Autodesk Inventor part; units mm, degrees
ref_plane "Arbeitsebene13" through (0, 0, 0) normal (0, 0, 1) x (1, 0, 0)
ref_plane "YZ Plane" through (0, 0, 0) normal (1, 0, 0) x (0, 1, 0)
ref_plane "XZ Plane" through (0, 0, 0) normal (0, 1, 0) x (-1, 0, 0)
sketch "Skizze1" plane through (0, 0, 0) normal (0, 0, 1) x (1, 0, 0)
  line L0 (0, 0) -> (30, 0)
  line L1 (0, 0) -> (0, 17.5)
  line L2 (0, 17.5) -> (3.5, 17.5)
  line L3 (3.5, 17.5) -> (3.5, 15.005)
  line L4 (3.5, 15.005) -> (6.6, 15.005)
  line L5 (6.6, 15.005) -> (6.6, 17.5)
  line L6 (6.6, 17.5) -> (13.5, 17.5)
  line L7 (13.5, 17.5) -> (13.5, 15.005)
  line L8 (13.5, 15.005) -> (16.6, 15.005)
  line L9 (16.6, 15.005) -> (16.6, 17.5)
  line L10 (16.6, 17.5) -> (30, 17.5)
  line L11 (30, 17.5) -> (30, 0)
  point P0 (13.5, 16.2525)
  dimension "d0" = 35
  dimension "d1" = 30.01
  dimension "d3" = 16.5
  dimension "d4" = 26.5
  dimension "d5" = 30
  dimension "d6" = 3.1
revolve "Umdrehung1" add sketch "Skizze1" angle 360 about axis through (0, 0, 0) along (1, 0, 0)
sketch "Skizze2" plane through (30, 0, 0) normal (1, 0, 0) x (0, 0, -1)
  circle A0 centre (0, 0) radius 17.5
hole "Bohrung1" at (30, 0, 0) direction (-1, 0, 0) diameter 25 depth 17.5 tip angle 118
fillet "Rundung1" radius 1 1 edges at (0, -17.5, 0)
fillet "Rundung2" radius 1 2 edges at (3.5, -15.005, 0) (13.5, -15.005, 0)
ref_plane "Arbeitsebene13" through (0, 0, 0) normal (0, 0, 1) x (1, 0, 0)
sketch "Skizze17" plane through (0, 0, 0) normal (0, 0, 1) x (1, 0, 0)
  line L0 (30, 12.5) -> (30, -12.5)
  point P0 (0, 0)
  point P1 (22, 0)
  dimension "d51" = 8
hole "Bohrung4" at (22, 0, 0) direction (0, 0, -1) diameter 5.98 end through all both
properties part number "Kolben" material "Stahl, galvanisiert"
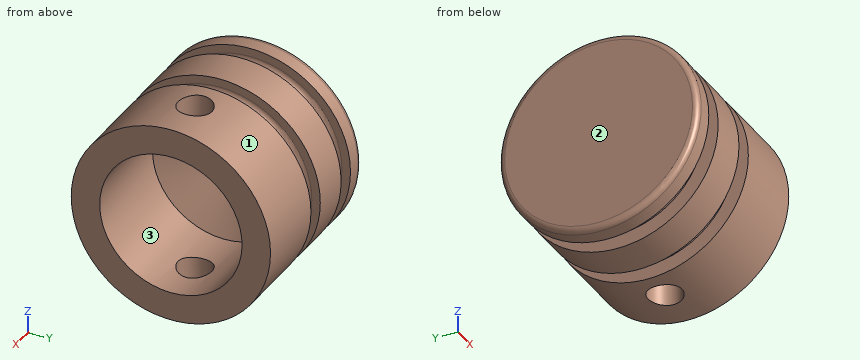
For this review, take the finished solid that the model builds, in its own axes (mm). Face numbers are marked on the shaded views. Coordinates: 2 decimals unless noted, no trailing zeros. Write each loop counter-clockwise with the first axis right and the second up, starting at its lowest first coordinate (ties: lowest second). Pieces come first, ordered by that corner, then holes. Notation, with made-up numbers: (51, -33.5) - (103, -33.5) arc R25 cw to (103, -12.5) - close; hole circle Ø1 at (-3.75, 80). An arc over 180 degrees is marked (long way). Answer in a Markdown table with one row per item. Add a question column.
Q1. For P1, Ø4, axis at x = 7.5, y = 7.5, coming from the -Z side; P2, Ø10, axis at y = -1, z = 1, coming from the +X side; P3, Ø8, axis at x = 22.5, y = -13, coming from the +Z side, all flat-tipped, find the tip position at first contact; note any pin that passes through.
Q2. We need section B-B, the plane x = 26. State the section outline as (y, z) points, and give its area (3 significant figures).
Q3. For probe 1 along X at (y, z) = (0, -15.9); probe 2 along X at (y, z) = (15.5, 6.5); probe 3 along Z at (x, y) = (16.25, 0) (3 decimals), list the stretches that pass through material, from the lowest coordinate up.
Q4. We need section A-A, the plane x = 22. State the section outline as (y, z) points.
Q5. Draft analysis for pull direction Y (two halves, no side actions). For the marked faces 1, 2 and 3, state which applies: +Y half, -Y half, draft (parallel to the pull), parting line (faces both ways), or undercut.
Answer list:
| question | item | result |
|---|---|---|
| 1 | P1 | stops at z = -16.61 |
| 1 | P2 | stops at x = 8.84 |
| 1 | P3 | stops at z = 15.01 |
| 2 | outline | circle Ø35 at (0, 0); hole circle Ø25 at (0, 0) |
| 2 | area | 471 mm2 |
| 3 | probe 1 | x = 0 to 3.51, 6.6 to 13.51, 16.6 to 19.01, 24.99 to 30 |
| 3 | probe 2 | x = 0.05 to 3.5, 6.6 to 13.5, 16.6 to 30 |
| 3 | probe 3 | z = -15.005 to -12.5, 12.5 to 15.005 |
| 4 | outline | (-2.99, -17.24) - (-2.99, -12.14) arc R12.5 cw to (-2.99, 12.14) - (-2.99, 17.24) arc R17.5 ccw to start; (2.99, -17.24) arc R17.5 ccw to (2.99, 17.24) - (2.99, 12.14) arc R12.5 cw to (2.99, -12.14) - close |
| 5 | face 1 | parting line |
| 5 | face 2 | draft |
| 5 | face 3 | undercut |
